from build123d import *

# Parameters (mm, degrees)
BOSS_EXTRUDE3_DEPTH = 8.5
SKETCH2_R           = 6.815
CUT_EXTRUDE1_DEPTH  = 862.437728783


with BuildPart() as part:
    # Sketch1 → Boss-Extrude3 (new body)
    with BuildSketch(Plane.XY):
        with BuildLine():
            ThreePointArc((395.972037607, 288.042278205), (410.873208436, 304.924541602), (388.360524278, 304.440019711))
            Line((388.360524278, 304.440019711), (-782.647332163, 9.376075193))
            ThreePointArc((-782.647332163, 9.376075193), (-802.796708748, -1.513309192), (-780.597372059, -7.1494))
            Line((-780.597372059, -7.1494), (-406.064833976, -7.1494))
            ThreePointArc((-406.064833976, -7.1494), (-395.672766052, -12.875746118), (-385.280698128, -7.1494))
            Line((-385.280698128, -7.1494), (-10.009831376, -7.1494))
            ThreePointArc((-10.009831376, -7.1494), (4.069984623, -11.891378206), (12.43312578, 0.388094335))
            Line((12.43312578, 0.388094335), (395.972037607, 288.042278205))
        make_face()
        with BuildLine():
            Line((-732.963454166, 7.1494), (280.120400531, 262.420546688))
            Line((280.120400531, 262.420546688), (-389.274490601, 9.913569288))
            ThreePointArc((-389.274490601, 9.913569288), (-397.771252158, 11.52949585), (-405.229196644, 7.1494))
            Line((-405.229196644, 7.1494), (-732.963454166, 7.1494))
        make_face(mode=Mode.SUBTRACT)
        with BuildLine():
            Line((355.529405997, 275.583804497), (3.528425073, 11.583068805))
            ThreePointArc((3.528425073, 11.583068805), (-3.75849008, 11.414643851), (-9.669090245, 7.1494))
            Line((-9.669090245, 7.1494), (-356.08902461, 7.1494))
            Line((-356.08902461, 7.1494), (355.529405997, 275.583804497))
        make_face(mode=Mode.SUBTRACT)
    extrude(amount=BOSS_EXTRUDE3_DEPTH)

    # Sketch2 → Cut-Extrude1 (cut, through all)
    with BuildSketch(Plane.XY.offset(8.5)):
        Circle(SKETCH2_R)
        with Locations((399.723044466, 299.74885191)):
            Circle(SKETCH2_R)
        with Locations((-395.609498981, 0)):
            Circle(SKETCH2_R)
        with Locations((-790.597372059, 0)):
            Circle(SKETCH2_R)
    extrude(amount=-CUT_EXTRUDE1_DEPTH, mode=Mode.SUBTRACT)


solid = part.part
CAD build for the part. Positions are in the model's coordinates, mm. A direction names the side the tool comes from. Coordinates: 2 decimals unless noted, no trailing zeros. Write each loop counter-clockwise with the first axis right and the second up, starting at its lowest first coordinate (ties: lowest second). Pieces come first, ordered by that corner, then holes. Notation, with made-up numbers: M -2,39 L 46,39 A25 ccw 46,63 Z; hole C 67,76 d10. An arc over 180 degrees is marked long. Answer as a JSON object with one key per item and string values. Group by question number.
1) Tool access for faces 1 (the face through (-198, 78, 8.5)), 2 (the face through (-5.26, 139.49, 4.19)): list every direction of +Z, -Z, +X, -X, +Y, -Y with a clear straight run to the whole face (end or side of a thin tool).
2) Saw through at B-B (y = 126). Write the cut outline in (x, z), plus the area to 3 significant figures.
3) Pin check, flat tips, straight feed: pin 1 Ø2.5 at (x, z) = (-648.5, 3) entering from -Y; pin 2 Ø4 at (x, z) = (-459, 1.5) entering from +Y; pin 3 Ø3 at (x, z) = (-204.5, 7) entering from +Y. Stop position of each tip, or through.
4) Wall check: line 1 (Y direction, x = -331.5, z = 2.5); line 2 (Y direction, x = -393, z = 1.5); line 3 (Y direction, x = -582, z = 4.25). Give the ranges that are in metal, low to high. Write a range as from..to.
5) Mould opens along X. For faces 3 (the face through (-198, 78, 0)), 4 (the face through (181.99, 145.43, 4.19)) say: +X half, -X half, draft (parallel to the pull), parting line (faces both ways), or undercut.
6) Saw through at D-D (z = 1.75). Write the cut outline in (x, y) (1 decimal), plus the area to 3 significant figures.
7) Saw through at C-C (x = -706). Write the cut outline in (y, z), plus the area to 3 significant figures.
8) Saw through at A-A (x = 119). Write the cut outline in (y, z), plus the area to 3 significant figures.
Values follow:
{
 "1": {"face 1": "+Z, +X, -X, +Y, -Y", "face 2": "+Z, -Z"},
 "2": {"outline": "M -319.81,0 L -261.29,0 L -261.29,8.5 L -319.81,8.5 Z; M -81.53,0 L -41.02,0 L -41.02,8.5 L -81.53,8.5 Z; M 156.08,0 L 179.92,0 L 179.92,8.5 L 156.08,8.5 Z", "area": "1,040 mm2"},
 "3": {"pin 1": "stops at y = -7.15", "pin 2": "stops at y = 91.43", "pin 3": "stops at y = 155.43"},
 "4": {"line 1": "y = -7.15..7.15, 16.42..31.71, 108.31..123.05", "line 2": "y = -12.58..-6.3, 6.3..11.42, 92.81..107.56", "line 3": "y = -7.15..7.15, 45.19..59.93"},
 "5": {"face 3": "draft", "face 4": "undercut"},
 "6": {"outline": "M -782.6,9.4 A12.3 ccw long -780.6,-7.1 L -406.1,-7.1 A12.3 ccw -385.3,-7.1 L -10,-7.1 A12.3 ccw 12.4,0.4 L 396,288 A12.3 ccw long 388.4,304.4 Z; hole C -790.6,0 d13.6; hole M -733,7.1 L -405.2,7.1 A12.3 cw -389.3,9.9 L 280.1,262.4 Z; hole C -395.6,0 d13.6; hole M -356.1,7.1 L -9.7,7.1 A12.3 cw 3.5,11.6 L 355.5,275.6 Z; hole C 0,0 d13.6; hole C 399.7,299.7 d13.6", "area": "46,500 mm2"},
 "7": {"outline": "M -7.15,0 L 7.15,0 L 7.15,8.5 L -7.15,8.5 Z; M 13.94,0 L 28.69,0 L 28.69,8.5 L 13.94,8.5 Z", "area": "247 mm2"},
 "8": {"outline": "M 80.31,0 L 98.19,0 L 98.19,8.5 L 80.31,8.5 Z; M 186.36,0 L 201.64,0 L 201.64,8.5 L 186.36,8.5 Z; M 221.82,0 L 236.57,0 L 236.57,8.5 L 221.82,8.5 Z", "area": "407 mm2"}
}
